Design review of the part built by this model. Coordinates are the model's own, in mm. Face numbers are marked on the shaded views. A direction names the side the tool comes from. Round coordinates to 2 decimals unless told otherwise and drop trailing zeros. Loops run counter-clockwise (first coordinate to the right, second up) from the corner with the lowest first, then second, coordinate; pieces in that order, holes last. Notation, with made-up numbers: (72.25, -5) - (121.25, -5) arc R23 cw to (121.25, 13) - close; hole circle Ø1 at (89.25, 69.5). An arc over 180 degrees is marked (long way). Use one line per item in the form item = value. Start each with the question number.
(1) The part is to be moulded in two halves that separate along Y. For the marked faces 3, 4 and 5, say which applies: released by +Y, released by -Y, zero draft, split by the parting line, or undercut.
(2) Wall thickness on probe 1 along X at (y, z) = (-0.25, 0.6); probe 2 along Z at (x, y) = (-4.5, -2.75); probe 3 along Y at (x, z) = (-2.75, 1.9): over which ranges is each line inside the solid? List them lowest first. Write a range as [from, to].
(3) We need section C-C, the plane z = 3.9. Write out the cut boundary in (x, y) (3 decimals).
(4) Machinability: for the marked faces 1 and 2, which of the approach directions +Z, -Z, +X, -X, +Y, -Y give a long, thin tool a straight path to every point of the face, cutting with its end or side? Answer none if there is none.
(5) For pin 1 (9 mm diameter, centred on x = 6, y = 3, fed in from -Z); pin 2 (2 mm diameter, centred on x = -0.5, y = 0, fed in from +Z), all flat-tipped, find the tip position at first contact; note any pin that passes through.
(6) We need section A-A, the plane z = 2.35. Write out the cut boundary in (x, y) (3 decimals), then the cut area to 3 significant figures.
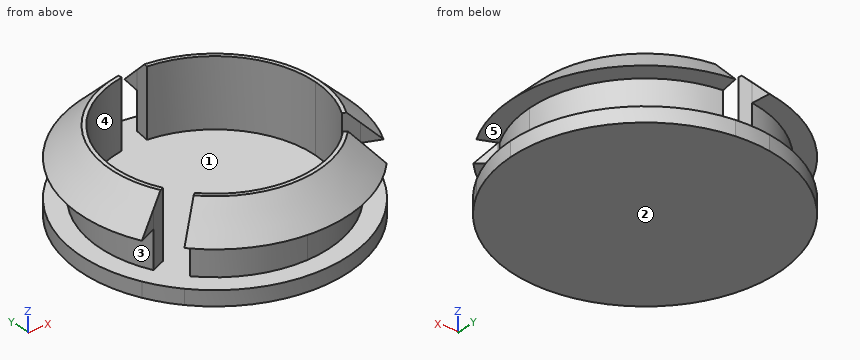
from build123d import *

# Parameters (mm, degrees)
F1_DEPTH = 1
F2_DEPTH = 5.5
F3_START = 3.5
F3_DEPTH = 2
F4_SIZE  = 1.99999


# Not quite as in the source:
# - a fillet or chamfer is up to 0.001 mm smaller than in the source, because OpenCascade refuses the exact size


with BuildPart() as f1:
    # F0 (on Top) → F1 (new body)
    with BuildSketch(Plane.XY):
        with BuildLine():
            ThreePointArc((6.675, 0), (4.9879380463, 4.4357749094), (0.7795396115, 6.6293244749))
            ThreePointArc((0.7795396115, 6.6293244749), (-0.0613991479, 6.6747176079), (-0.9013605528, 6.6138622721))
            ThreePointArc((-0.9013605528, 6.6138622721), (-5.9267464923, 3.0707166942), (-5.9228974074, -3.0781343864))
            ThreePointArc((-5.9228974074, -3.0781343864), (-5.4750931221, -3.8182430914), (-4.9353373694, -4.4942263016))
            ThreePointArc((-4.9353373694, -4.4942263016), (-2.6978384344, -6.1055133103), (0, -6.675))
            ThreePointArc((0, -6.675), (2.6066720123, -6.1449886916), (4.7993917719, -4.6391231521))
            ThreePointArc((4.7993917719, -4.6391231521), (5.3679142179, -3.9675082796), (5.8431534535, -3.2269463459))
            ThreePointArc((5.8431534535, -3.2269463459), (6.4636937699, -1.6662196281), (6.675, 0))
        make_face()
        with BuildLine():
            Line((-5.9228974074, -3.0781343864), (-6.849796149, -3.4620684161))
            ThreePointArc((-6.849796149, -3.4620684161), (-6.3438696558, -4.3198313381), (-5.7311395238, -5.1048667718))
            Line((-5.7311395238, -5.1048667718), (-4.9353373694, -4.4942263016))
            ThreePointArc((-4.9353373694, -4.4942263016), (-5.4750931221, -3.8182430914), (-5.9228974074, -3.0781343864))
        make_face()
        with BuildLine():
            Line((-6.849796149, -3.4620684161), (-8.0074646458, -3.9415904082))
            ThreePointArc((-8.0074646458, -3.9415904082), (-7.4289702623, -4.9463143695), (-6.7251178515, -5.8675731681))
            Line((-6.7251178515, -5.8675731681), (-5.7311395238, -5.1048667718))
            ThreePointArc((-5.7311395238, -5.1048667718), (-6.3438696558, -4.3198313381), (-6.849796149, -3.4620684161))
        make_face()
        with BuildLine():
            Line((0.9100766885, 7.6208520141), (1.0732446043, 8.8602353817))
            ThreePointArc((1.0732446043, 8.8602353817), (-0.0613988555, 8.9247888031), (-1.1950467583, 8.8446304754))
            Line((-1.1950467583, 8.8446304754), (-1.0318879198, 7.6053160566))
            ThreePointArc((-1.0318879198, 7.6053160566), (-0.0613989862, 7.6747544042), (0.9100766885, 7.6208520141))
        make_face()
        with BuildLine():
            Line((-1.0318879198, 7.6053160566), (-1.1950467583, 8.8446304754))
            ThreePointArc((-1.1950467583, 8.8446304754), (-7.8767642568, 4.196690344), (-8.0074646458, -3.9415904082))
            Line((-8.0074646458, -3.9415904082), (-6.849796149, -3.4620684161))
            ThreePointArc((-6.849796149, -3.4620684161), (-6.7935252783, 3.5712237809), (-1.0318879198, 7.6053160566))
        make_face()
        with BuildLine():
            ThreePointArc((-6.7251178515, -5.8675731681), (-3.6937470456, -8.1247681667), (0, -8.925))
            Line((0, -8.925), (0, -7.675))
            ThreePointArc((0, -7.675), (-3.1405232467, -7.0030521015), (-5.7311395238, -5.1048667718))
            Line((-5.7311395238, -5.1048667718), (-6.7251178515, -5.8675731681))
        make_face()
        with BuildLine():
            ThreePointArc((0, -8.925), (3.6032793864, -8.1652925645), (6.5931272563, -6.0155047986))
            Line((6.5931272563, -6.0155047986), (5.597241272, -5.2513346059))
            ThreePointArc((5.597241272, -5.2513346059), (3.0497239137, -7.043068156), (0, -7.675))
            Line((0, -7.675), (0, -8.925))
        make_face()
        with BuildLine():
            ThreePointArc((6.5931272563, -6.0155047986), (7.3257881446, -5.0978871172), (7.9316419101, -4.0920265895))
            Line((7.9316419101, -4.0920265895), (6.7720820443, -3.6117211667))
            ThreePointArc((6.7720820443, -3.6117211667), (6.2387597231, -4.4702910551), (5.597241272, -5.2513346059))
            Line((5.597241272, -5.2513346059), (6.5931272563, -6.0155047986))
        make_face()
        with BuildLine():
            ThreePointArc((7.9316419101, -4.0920265895), (8.6731058176, -2.1054359349), (8.925, 0))
            ThreePointArc((8.925, 0), (6.679608263, 5.9193292233), (1.0732446043, 8.8602353817))
            Line((1.0732446043, 8.8602353817), (0.9100766885, 7.6208520141))
            ThreePointArc((0.9100766885, 7.6208520141), (5.7397937064, 5.0951342679), (7.675, 0))
            ThreePointArc((7.675, 0), (7.4458496725, -1.8614369866), (6.7720820443, -3.6117211667))
            Line((6.7720820443, -3.6117211667), (7.9316419101, -4.0920265895))
        make_face()
        with BuildLine():
            ThreePointArc((5.597241272, -5.2513346059), (6.2387597231, -4.4702910551), (6.7720820443, -3.6117211667))
            Line((6.7720820443, -3.6117211667), (5.8431534535, -3.2269463459))
            ThreePointArc((5.8431534535, -3.2269463459), (5.3679142179, -3.9675082796), (4.7993917719, -4.6391231521))
            Line((4.7993917719, -4.6391231521), (5.597241272, -5.2513346059))
        make_face()
        with BuildLine():
            Line((0.7795396115, 6.6293244749), (0.9100766885, 7.6208520141))
            ThreePointArc((0.9100766885, 7.6208520141), (-0.0613989862, 7.6747544042), (-1.0318879198, 7.6053160566))
            Line((-1.0318879198, 7.6053160566), (-0.9013605528, 6.6138622721))
            ThreePointArc((-0.9013605528, 6.6138622721), (-0.0613991479, 6.6747176079), (0.7795396115, 6.6293244749))
        make_face()
    extrude(amount=F1_DEPTH)

    # F0 (on Top) → F2 (join)
    with BuildSketch(Plane.XY):
        with BuildLine():
            Line((-0.9013605528, 6.6138622721), (-1.0318879198, 7.6053160566))
            ThreePointArc((-1.0318879198, 7.6053160566), (-6.7935252783, 3.5712237809), (-6.849796149, -3.4620684161))
            Line((-6.849796149, -3.4620684161), (-5.9228974074, -3.0781343864))
            ThreePointArc((-5.9228974074, -3.0781343864), (-5.9267464923, 3.0707166942), (-0.9013605528, 6.6138622721))
        make_face()
        with BuildLine():
            ThreePointArc((7.675, 0), (5.7397937064, 5.0951342679), (0.9100766885, 7.6208520141))
            Line((0.9100766885, 7.6208520141), (0.7795396115, 6.6293244749))
            ThreePointArc((0.7795396115, 6.6293244749), (4.9879380463, 4.4357749094), (6.675, 0))
            ThreePointArc((6.675, 0), (6.4636937699, -1.6662196281), (5.8431534535, -3.2269463459))
            Line((5.8431534535, -3.2269463459), (6.7720820443, -3.6117211667))
            ThreePointArc((6.7720820443, -3.6117211667), (7.4458496725, -1.8614369866), (7.675, 0))
        make_face()
        with BuildLine():
            ThreePointArc((-5.7311395238, -5.1048667718), (-3.1405232467, -7.0030521015), (0, -7.675))
            Line((0, -7.675), (0, -6.675))
            ThreePointArc((0, -6.675), (-2.6978384344, -6.1055133103), (-4.9353373694, -4.4942263016))
            Line((-4.9353373694, -4.4942263016), (-5.7311395238, -5.1048667718))
        make_face()
        with BuildLine():
            ThreePointArc((0, -7.675), (3.0497239137, -7.043068156), (5.597241272, -5.2513346059))
            Line((5.597241272, -5.2513346059), (4.7993917719, -4.6391231521))
            ThreePointArc((4.7993917719, -4.6391231521), (2.6066720123, -6.1449886916), (0, -6.675))
            Line((0, -6.675), (0, -7.675))
        make_face()
    extrude(amount=F2_DEPTH)

    # F0 (on Top) → F3 (join)
    with BuildSketch(Plane.XY.offset(F3_START)):
        with BuildLine():
            Line((-1.0318879198, 7.6053160566), (-1.1950467583, 8.8446304754))
            ThreePointArc((-1.1950467583, 8.8446304754), (-7.8767642568, 4.196690344), (-8.0074646458, -3.9415904082))
            Line((-8.0074646458, -3.9415904082), (-6.849796149, -3.4620684161))
            ThreePointArc((-6.849796149, -3.4620684161), (-6.7935252783, 3.5712237809), (-1.0318879198, 7.6053160566))
        make_face()
        with BuildLine():
            ThreePointArc((7.9316419101, -4.0920265895), (8.6731058176, -2.1054359349), (8.925, 0))
            ThreePointArc((8.925, 0), (6.679608263, 5.9193292233), (1.0732446043, 8.8602353817))
            Line((1.0732446043, 8.8602353817), (0.9100766885, 7.6208520141))
            ThreePointArc((0.9100766885, 7.6208520141), (5.7397937064, 5.0951342679), (7.675, 0))
            ThreePointArc((7.675, 0), (7.4458496725, -1.8614369866), (6.7720820443, -3.6117211667))
            Line((6.7720820443, -3.6117211667), (7.9316419101, -4.0920265895))
        make_face()
        with BuildLine():
            ThreePointArc((0, -8.925), (3.6032793864, -8.1652925645), (6.5931272563, -6.0155047986))
            Line((6.5931272563, -6.0155047986), (5.597241272, -5.2513346059))
            ThreePointArc((5.597241272, -5.2513346059), (3.0497239137, -7.043068156), (0, -7.675))
            Line((0, -7.675), (0, -8.925))
        make_face()
        with BuildLine():
            ThreePointArc((-6.7251178515, -5.8675731681), (-3.6937470456, -8.1247681667), (0, -8.925))
            Line((0, -8.925), (0, -7.675))
            ThreePointArc((0, -7.675), (-3.1405232467, -7.0030521015), (-5.7311395238, -5.1048667718))
            Line((-5.7311395238, -5.1048667718), (-6.7251178515, -5.8675731681))
        make_face()
    extrude(amount=F3_DEPTH)

    # F4 (size 2 in the source; OpenCascade refuses exactly that, so slightly less here)
    f4_edges = [f1.edges().sort_by_distance(p)[0] for p in [
        (-7.876764, 4.19669, 5.5),
        (-0.099128, -8.924449, 5.5),
        (7.887475, 4.176525, 5.5),
    ]]
    chamfer(f4_edges, length=F4_SIZE)


solid = f1.part
Data:
q1.face_3 = split by the parting line
q1.face_4 = undercut
q1.face_5 = zero draft
q2.probe_1 = [-8.92, 8.92]
q2.probe_2 = [0, 1]
q2.probe_3 = [-7.17, -6.08], [6.08, 7.17]
q3.outline = (-7.637, -3.788) - (-5.923, -3.078) arc R6.675 cw to (-0.901, 6.614) - (-1.143, 8.448) arc R8.525 ccw to start; (-6.407, -5.624) arc R8.525 ccw to (6.275, -5.771) - (4.799, -4.639) arc R6.675 cw to (-4.935, -4.494) - close; (0.78, 6.629) arc R6.675 cw to (5.843, -3.227) - (7.561, -3.938) arc R8.525 ccw to (1.021, 8.464) - close
q4.face_1 = none
q4.face_2 = -Z, +X, -X, +Y, -Y
q5.pin_1 = 0
q5.pin_2 = 1
q6.outline = (-6.85, -3.462) - (-5.923, -3.078) arc R6.675 cw to (-0.901, 6.614) - (-1.032, 7.605) arc R7.675 ccw to start; (-5.731, -5.105) arc R7.675 ccw to (5.597, -5.251) - (4.799, -4.639) arc R6.675 cw to (-4.935, -4.494) - close; (0.78, 6.629) arc R6.675 cw to (5.843, -3.227) - (6.772, -3.612) arc R7.675 ccw to (0.91, 7.621) - close
q6.area = 39.5 mm^2
